Could you check a few things on this model? Use its own coordinates, in mm. A direction names the side the tool comes from. Coordinates: 2 decimals unless noted, no trailing zeros. Order: outer loops, then holes, each group sorted by start corner. A loop starts at its lowest first (then second) coordinate and runs counter-clockwise, first axis right, second up. Notation, with made-up numbers: (78, 61.25) -> (120, 61.25) arc R9 cw to (120, 76.25) -> close; hole circle Ø3 at (-36.5, -34). An arc over 180 degrees is marked (long way). Use a Markdown table: item, result. Add a question column.
1) Will these pins go through, and if not, where does the flat tip stop? pin 1 Ø2 at (y, z) = (-3, 0.5) entering from -X; pin 2 Ø1.5 at (x, z) = (5.5, 1.5) entering from -Y; pin 3 Ø1.5 at (y, z) = (-14, 0.5) entering from -X.
2) Thinking about a two-plate mould opening in X: for faces 1 (the cylindrical face through (-8.4, -0.07, 1.77)), 2 (the cylindrical face through (-54, 0, 2)), 3 (the flat face through (53, 7.555, 2)), which applies, +X half, -X half, draft (parallel to the pull), parting line (faces both ways), or undercut?
3) If we section it at C-C (y = -7): Write out the boundary of the cut face in (x, z), plus the area to 3 significant figures.
4) If we section it at D-D (x = 25): Write out the boundary of the cut face in (y, z).
5) If I drill on L1, parallel to X at y = 0, z = 1.2; L2, parallel to Y at x = -10, z = 2; L3, parallel to Y at x = -37, z = 0.25, over which ranges is the centre line in solid material (lowest first)? Write a range as [from, to].
6) If we section it at B-B (x = -10): Write out the boundary of the cut face in (y, z).
7) Which directions (+Z, -Z, +X, -X, +Y, -Y) give clear straight access to the entire face, cutting with the end or side of a thin tool? Please do faces 4 (the flat face through (-26, -4, 2)), 5 (the flat face through (-23, 4, 2)), 6 (the flat face through (6, -5, 0)).
8) If we section it at A-A (z = 2.7): Write out the boundary of the cut face in (x, y), plus the area to 3 significant figures.
```python
from build123d import *

# Parameters (mm, degrees)
F1_DEPTH = 3.5
F3_DEPTH = 3.501


# Not quite as in the source:
# - a feature names something its author has since deleted; it is built from what else it names


with BuildPart() as f1:
    # F0 (on Top) → F1 (new body)
    with BuildSketch(Plane.XY):
        with BuildLine():
            ThreePointArc((-50, 4), (-54, 0), (-50, -4))
            Line((-50, -4), (-50, 4))
        make_face()
        with BuildLine():
            Line((-50, 4), (-50, -4))
            ThreePointArc((-50, -4), (-47.1715728753, -2.8284271247), (-46, 0))
            ThreePointArc((-46, 0), (-47.1715728753, 2.8284271247), (-50, 4))
        make_face()
        with BuildLine():
            Line((-50, -4), (-2.1705369066, -4))
            ThreePointArc((-2.1705369066, -4), (-4.496147737, -0.1398594601), (-6.2767977228, 4))
            Line((-6.2767977228, 4), (-50, 4))
            ThreePointArc((-50, 4), (-47.1715728753, 2.8284271247), (-46, 0))
            ThreePointArc((-46, 0), (-47.1715728753, -2.8284271247), (-50, -4))
        make_face()
        with BuildLine():
            Line((-2.1705369066, -4), (8.5147968103, -4))
            ThreePointArc((8.5147968103, -4), (6.5521066164, -2.1007939556), (4.8068842373, 0))
            ThreePointArc((4.8068842373, 0), (3.4991426783, 1.9433902318), (2.3778443952, 4))
            Line((2.3778443952, 4), (-6.2767977228, 4))
            ThreePointArc((-6.2767977228, 4), (-4.496147737, -0.1398594601), (-2.1705369066, -4))
        make_face()
        with BuildLine():
            ThreePointArc((53.4299716908, -2.0579830418), (51.9707952498, -3.4807996328), (50, -4))
            Line((50, -4), (41.4852031897, -4))
            ThreePointArc((41.4852031897, -4), (25, -10.1547594742), (8.5147968103, -4))
            Line((8.5147968103, -4), (-2.1705369066, -4))
            ThreePointArc((-2.1705369066, -4), (26.1573251317, -18.1345540838), (53.4299716908, -2.0579830418))
        make_face()
        with BuildLine():
            Line((41.4852031897, -4), (50, -4))
            ThreePointArc((50, -4), (47.1715728753, -2.8284271247), (46, 0))
            Line((46, 0), (45.1931157627, 0))
            ThreePointArc((45.1931157627, 0), (43.4478933836, -2.1007939556), (41.4852031897, -4))
        make_face()
        with BuildLine():
            ThreePointArc((46, 0), (47.1715728753, -2.8284271247), (50, -4))
            Line((50, -4), (50, 0))
            Line((50, 0), (46, 0))
        make_face()
        with BuildLine():
            Line((50, 0), (50, -4))
            ThreePointArc((50, -4), (51.9707952498, -3.4807996328), (53.4299716908, -2.0579830418))
            ThreePointArc((53.4299716908, -2.0579830418), (53.8548597097, -1.0677343389), (54, 0))
            ThreePointArc((54, 0), (52.8284271247, 2.8284271247), (50, 4))
            Line((50, 4), (50, 0))
        make_face()
        with BuildLine():
            Line((46, 0), (50, 0))
            Line((50, 0), (50, 4))
            ThreePointArc((50, 4), (48.0292047387, 3.4807996262), (46.5700282955, 2.0579830189))
            ThreePointArc((46.5700282955, 2.0579830189), (46.1451402867, 1.067734326), (46, 0))
        make_face()
        with BuildLine():
            ThreePointArc((46.5700282955, 2.0579830189), (48.0292047387, 3.4807996262), (50, 4))
            Line((50, 4), (47.6221556048, 4))
            ThreePointArc((47.6221556048, 4), (47.1174170499, 3.0174382017), (46.5700282955, 2.0579830189))
        make_face()
        with BuildLine():
            Line((45.1931157627, 0), (46, 0))
            ThreePointArc((46, 0), (46.1451402867, 1.067734326), (46.5700282955, 2.0579830189))
            ThreePointArc((46.5700282955, 2.0579830189), (45.9069097174, 1.0120390952), (45.1931157627, 0))
        make_face()
        with BuildLine():
            ThreePointArc((54, 0), (53.8548597097, -1.0677343389), (53.4299716908, -2.0579830418))
            ThreePointArc((53.4299716908, -2.0579830418), (55.7469814085, 2.5959196207), (57.3080045365, 7.5548056666))
            Line((57.3080045365, 7.5548056666), (49.0277132816, 7.5548056666))
            ThreePointArc((49.0277132816, 7.5548056666), (48.3925570986, 5.7506650728), (47.6221556048, 4))
            Line((47.6221556048, 4), (50, 4))
            ThreePointArc((50, 4), (52.8284271247, 2.8284271247), (54, 0))
        make_face()
    extrude(amount=F1_DEPTH)

    # F2 (on face) → F3 (cut, through all)
    with BuildSketch(Plane.XY.offset(3.5)):
        with BuildLine():
            ThreePointArc((-48.4, 0), (-48.8686291501, 1.1313708499), (-50, 1.6))
            Line((-50, 1.6), (-50, 0))
            Line((-50, 0), (-48.4, 0))
        make_face()
        with BuildLine():
            Line((-50, 0), (-50, 1.6))
            ThreePointArc((-50, 1.6), (-51.6, 0), (-50, -1.6))
            Line((-50, -1.6), (-50, 0))
        make_face()
        with BuildLine():
            ThreePointArc((-8.4, 0), (-10, 1.6), (-11.6, 0))
            ThreePointArc((-11.6, 0), (-10, -1.6), (-8.4, 0))
        make_face()
        with BuildLine():
            Line((-48.4, 0), (-50, 0))
            Line((-50, 0), (-50, -1.6))
            ThreePointArc((-50, -1.6), (-48.8686291501, -1.1313708499), (-48.4, 0))
        make_face()
    extrude(amount=-F3_DEPTH, mode=Mode.SUBTRACT)


solid = f1.part
```
Answer sheet:
| question | item | result |
|---|---|---|
| 1 | pin 1 | x = -53.46 |
| 1 | pin 2 | y = -12.34 |
| 1 | pin 3 | x = 7.65 |
| 2 | face 1 | undercut |
| 2 | face 2 | -X half |
| 2 | face 3 | draft |
| 3 | outline | (0.2, 0) -> (12.8, 0) -> (12.8, 3.5) -> (0.2, 3.5) -> close; (37.2, 0) -> (49.8, 0) -> (49.8, 3.5) -> (37.2, 3.5) -> close |
| 3 | area | 88.3 mm2 |
| 4 | outline | (-18.15, 0) -> (-10.15, 0) -> (-10.15, 3.5) -> (-18.15, 3.5) -> close |
| 5 | L1 | [-54, -51.6], [-48.4, -11.6], [-8.4, 4.81], [45.19, 54.57] |
| 5 | L2 | [-4, -1.6], [1.6, 4] |
| 5 | L3 | [-4, 4] |
| 6 | outline | (-4, 0) -> (-1.6, 0) -> (-1.6, 3.5) -> (-4, 3.5) -> close; (1.6, 0) -> (4, 0) -> (4, 3.5) -> (1.6, 3.5) -> close |
| 7 | face 4 | +Z, -Z, -X, -Y |
| 7 | face 5 | +Z, -Z, -X, +Y |
| 7 | face 6 | -Z, +X, -X, +Y, -Y |
| 8 | outline | (-50, -4) -> (-2.17, -4) arc R33.15 ccw to (57.31, 7.55) -> (49.03, 7.55) arc R25.15 cw to (2.38, 4) -> (-50, 4) arc R4 ccw to start; hole circle Ø3.2 at (-50, 0); hole circle Ø3.2 at (-10, 0) |
| 8 | area | 956 mm2 |
